from build123d import *

# Parameters (mm, degrees)
SKETCH_1_W          = 52
SKETCH_1_H          = 25
SKETCH_1_R          = 1.5
SKETCH_1_R_2        = 4
EXTRUDE_1_DEPTH     = 2
SKETCH_2_W          = 2
SKETCH_2_H          = 25
EXTRUDE_2_DEPTH     = 64.5
CUT_EXTRUDE_2_REACH = 91.001
SKETCH_3_R          = 1.5
FILLET_1_R          = 3


with BuildPart() as part:
    # 草图1 → 凸台-拉伸1 (new body)
    with BuildSketch(Plane(origin=(0, 0, 0), x_dir=(1, 0, 0), z_dir=(0, 1, 0))):
        with Locations((26, -12.5)):
            Rectangle(SKETCH_1_W, SKETCH_1_H)
        with Locations(Location((44.6, -12.5, 0), (0, 0, 270))):
            Circle(SKETCH_1_R, mode=Mode.SUBTRACT)
        with Locations(Location((26, -12.5, 0), (0, 0, 270))):
            Circle(SKETCH_1_R_2, mode=Mode.SUBTRACT)
        with Locations(Location((26, -19.5, 0), (0, 0, 270))):
            Circle(SKETCH_1_R, mode=Mode.SUBTRACT)
        with Locations(Location((19, -12.5, 0), (0, 0, 270))):
            Circle(SKETCH_1_R, mode=Mode.SUBTRACT)
        with Locations(Location((26, -5.5, 0), (0, 0, 270))):
            Circle(SKETCH_1_R, mode=Mode.SUBTRACT)
        with Locations(Location((33, -12.5, 0), (0, 0, 270))):
            Circle(SKETCH_1_R, mode=Mode.SUBTRACT)
        with Locations(Location((7.4, -12.5, 0), (0, 0, 90))):
            Circle(SKETCH_1_R, mode=Mode.SUBTRACT)
    extrude(amount=EXTRUDE_1_DEPTH)

    # 草图2 → 凸台-拉伸2 (add)
    with BuildSketch(Plane(origin=(0, 0, 0), x_dir=(1, 0, 0), z_dir=(0, 1, 0))):
        with Locations((-1, -12.5)):
            Rectangle(SKETCH_2_W, SKETCH_2_H)
        with Locations((53, -12.5)):
            Rectangle(SKETCH_2_W, SKETCH_2_H)
    extrude(amount=EXTRUDE_2_DEPTH)

    # 切除-拉伸2: up to this face of the body (flat: up to its plane)
    cut_extrude_2_end = Plane(part.part.faces().sort_by_distance((54, 32.25, 12.5))[0])
    # 草图3 → 切除-拉伸2 (cut, up to the picked face)
    with BuildSketch(Plane.ZY.offset(2), mode=Mode.PRIVATE) as cut_extrude_2_sk1:
        with BuildLine():
            Line((0, 64.5), (0, 52))
            ThreePointArc((0, 52), (3.661165235, 60.838834765), (12.5, 64.5))
            Line((12.5, 64.5), (0, 64.5))
        make_face()
    cut_extrude_2_tool1 = split(extrude(cut_extrude_2_sk1.sketch, amount=-CUT_EXTRUDE_2_REACH, mode=Mode.PRIVATE), bisect_by=cut_extrude_2_end, keep=Keep.BOTH, mode=Mode.PRIVATE)
    # 草图3 → 切除-拉伸2 (cut, up to the picked face)
    with BuildSketch(Plane.ZY.offset(2), mode=Mode.PRIVATE) as cut_extrude_2_sk2:
        with BuildLine():
            Line((25, 64.5), (12.5, 64.5))
            ThreePointArc((12.5, 64.5), (21.338834765, 60.838834765), (25, 52))
            Line((25, 52), (25, 64.5))
        make_face()
    cut_extrude_2_tool2 = split(extrude(cut_extrude_2_sk2.sketch, amount=-CUT_EXTRUDE_2_REACH, mode=Mode.PRIVATE), bisect_by=cut_extrude_2_end, keep=Keep.BOTH, mode=Mode.PRIVATE)
    # 草图3 → 切除-拉伸2 (cut, up to the picked face)
    with BuildSketch(Plane.ZY.offset(2), mode=Mode.PRIVATE) as cut_extrude_2_sk3:
        with BuildLine():
            ThreePointArc((16.5, 52), (12.5, 56), (8.5, 52))
            Line((8.5, 52), (16.5, 52))
        make_face()
    cut_extrude_2_tool3 = split(extrude(cut_extrude_2_sk3.sketch, amount=-CUT_EXTRUDE_2_REACH, mode=Mode.PRIVATE), bisect_by=cut_extrude_2_end, keep=Keep.BOTH, mode=Mode.PRIVATE)
    # 草图3 → 切除-拉伸2 (cut, up to the picked face)
    with BuildSketch(Plane.ZY.offset(2), mode=Mode.PRIVATE) as cut_extrude_2_sk4:
        with BuildLine():
            Line((16.5, 52), (8.5, 52))
            ThreePointArc((8.5, 52), (12.5, 48), (16.5, 52))
        make_face()
    cut_extrude_2_tool4 = split(extrude(cut_extrude_2_sk4.sketch, amount=-CUT_EXTRUDE_2_REACH, mode=Mode.PRIVATE), bisect_by=cut_extrude_2_end, keep=Keep.BOTH, mode=Mode.PRIVATE)
    # 草图3 → 切除-拉伸2 (cut, up to the picked face)
    with BuildSketch(Plane.ZY.offset(2), mode=Mode.PRIVATE) as cut_extrude_2_sk5:
        with BuildLine():
            ThreePointArc((16.5, 52), (12.5, 56), (8.5, 52))
            Line((8.5, 52), (16.5, 52))
        make_face()
    cut_extrude_2_tool5 = split(extrude(cut_extrude_2_sk5.sketch, amount=-CUT_EXTRUDE_2_REACH, mode=Mode.PRIVATE), bisect_by=cut_extrude_2_end, keep=Keep.BOTH, mode=Mode.PRIVATE)
    # 草图3 → 切除-拉伸2 (cut, up to the picked face)
    with BuildSketch(Plane.ZY.offset(2), mode=Mode.PRIVATE) as cut_extrude_2_sk6:
        with BuildLine():
            Line((16.5, 52), (8.5, 52))
            ThreePointArc((8.5, 52), (12.5, 48), (16.5, 52))
        make_face()
    cut_extrude_2_tool6 = split(extrude(cut_extrude_2_sk6.sketch, amount=-CUT_EXTRUDE_2_REACH, mode=Mode.PRIVATE), bisect_by=cut_extrude_2_end, keep=Keep.BOTH, mode=Mode.PRIVATE)
    # 草图3 → 切除-拉伸2 (cut, up to the picked face)
    with BuildSketch(Plane.ZY.offset(2), mode=Mode.PRIVATE) as cut_extrude_2_sk7:
        with Locations((12.5, 45)):
            Circle(SKETCH_3_R)
    cut_extrude_2_tool7 = split(extrude(cut_extrude_2_sk7.sketch, amount=-CUT_EXTRUDE_2_REACH, mode=Mode.PRIVATE), bisect_by=cut_extrude_2_end, keep=Keep.BOTH, mode=Mode.PRIVATE)
    # 草图3 → 切除-拉伸2 (cut, up to the picked face)
    with BuildSketch(Plane.ZY.offset(2), mode=Mode.PRIVATE) as cut_extrude_2_sk8:
        with Locations((12.5, 59)):
            Circle(SKETCH_3_R)
    cut_extrude_2_tool8 = split(extrude(cut_extrude_2_sk8.sketch, amount=-CUT_EXTRUDE_2_REACH, mode=Mode.PRIVATE), bisect_by=cut_extrude_2_end, keep=Keep.BOTH, mode=Mode.PRIVATE)
    # 草图3 → 切除-拉伸2 (cut, up to the picked face)
    with BuildSketch(Plane.ZY.offset(2), mode=Mode.PRIVATE) as cut_extrude_2_sk9:
        with Locations((5.5, 52)):
            Circle(SKETCH_3_R)
    cut_extrude_2_tool9 = split(extrude(cut_extrude_2_sk9.sketch, amount=-CUT_EXTRUDE_2_REACH, mode=Mode.PRIVATE), bisect_by=cut_extrude_2_end, keep=Keep.BOTH, mode=Mode.PRIVATE)
    # 草图3 → 切除-拉伸2 (cut, up to the picked face)
    with BuildSketch(Plane.ZY.offset(2), mode=Mode.PRIVATE) as cut_extrude_2_sk10:
        with Locations((19.5, 52)):
            Circle(SKETCH_3_R)
    cut_extrude_2_tool10 = split(extrude(cut_extrude_2_sk10.sketch, amount=-CUT_EXTRUDE_2_REACH, mode=Mode.PRIVATE), bisect_by=cut_extrude_2_end, keep=Keep.BOTH, mode=Mode.PRIVATE)
    add(cut_extrude_2_tool1.solids().sort_by(Axis((-2, 61.707901, 2.792099), (1, 0, 0)))[0], mode=Mode.SUBTRACT)
    add(cut_extrude_2_tool2.solids().sort_by(Axis((-2, 61.707901, 22.207901), (1, 0, 0)))[0], mode=Mode.SUBTRACT)
    add(cut_extrude_2_tool3.solids().sort_by(Axis((-2, 53.697653, 12.5), (1, 0, 0)))[0], mode=Mode.SUBTRACT)
    add(cut_extrude_2_tool4.solids().sort_by(Axis((-2, 50.302347, 12.5), (1, 0, 0)))[0], mode=Mode.SUBTRACT)
    add(cut_extrude_2_tool5.solids().sort_by(Axis((-2, 53.697653, 12.5), (1, 0, 0)))[0], mode=Mode.SUBTRACT)
    add(cut_extrude_2_tool6.solids().sort_by(Axis((-2, 50.302347, 12.5), (1, 0, 0)))[0], mode=Mode.SUBTRACT)
    add(cut_extrude_2_tool7.solids().sort_by(Axis((-2, 45, 12.5), (1, 0, 0)))[0], mode=Mode.SUBTRACT)
    add(cut_extrude_2_tool8.solids().sort_by(Axis((-2, 59, 12.5), (1, 0, 0)))[0], mode=Mode.SUBTRACT)
    add(cut_extrude_2_tool9.solids().sort_by(Axis((-2, 52, 5.5), (1, 0, 0)))[0], mode=Mode.SUBTRACT)
    add(cut_extrude_2_tool10.solids().sort_by(Axis((-2, 52, 19.5), (1, 0, 0)))[0], mode=Mode.SUBTRACT)

    # 圆角1
    fillet_1_edges = [part.edges().sort_by_distance(p)[0] for p in [
        (52, 2, 12.5),
        (0, 2, 12.5),
        (-2, 0, 12.5),
        (54, 0, 12.5),
    ]]
    fillet(fillet_1_edges, radius=FILLET_1_R)


solid = part.part
Geometry: final body of the model. Coordinates: model frame, mm. A direction names the side the tool comes from. Coordinates: 2 decimals unless noted, no trailing zeros. Write each loop counter-clockwise with the first axis right and the second up, starting at its lowest first coordinate (ties: lowest second). Pieces come first, ordered by that corner, then holes. Notation, with made-up numbers: (80, -17) - (138, -17) arc R17 cw to (138, 7) - close; hole circle Ø7 at (65.25, 81). An arc over 180 degrees is marked (long way). Return JSON: item names as keys, results as strings.
Item 1: Section query A-A (x = 26). Output: boundary loops of the cut face in (y, z), and give its area (3 significant figures).
Completed:
{"outline": "(0, 0) - (2, 0) - (2, 4) - (0, 4) - close; (0, 7) - (2, 7) - (2, 8.5) - (0, 8.5) - close; (0, 16.5) - (2, 16.5) - (2, 18) - (0, 18) - close; (0, 21) - (2, 21) - (2, 25) - (0, 25) - close", "area": "22.0 mm2"}
Item 2: Pull-direction query (Y, two-part tool) for faces 3 (the face through (-1, 51.1, 18.3)), 4 (the face through (27.487, 0.986, 5.305)), 5 (the face through (-1.14, 0.9, 12.32)); classes: +Y half, -Y half, draft (parallel to the pull), parting line (faces both ways), or undercut.
Completed:
{"face 3": "undercut", "face 4": "draft", "face 5": "-Y half"}
Item 3: Reachability of faces 1 (the face through (31, 2, 12)), 2 (the face through (26, 1, 25)) from +Z, -Z, +X, -X, +Y, -Y: full face, straight path, thin tool, end or side. Return the list, or none.
Completed:
{"face 1": "+Z, -Z, +Y", "face 2": "+Z, +X, -X, +Y, -Y"}
Item 4: Line query: L1, parallel to X at y = 26.5, z = 6.5; L2, parallel to Y at x = -1.1, z = 12.5; L3, parallel to X at y = 1.25, z = 12.5. Output: solid intervals per line, ascending.
Completed:
{"L1": "x = -2 to 0, 52 to 54", "L2": "y = 0.86 to 43.5, 46.5 to 48, 56 to 57.5, 60.5 to 64.5", "L3": "x = -1.44 to 5.9, 8.9 to 17.5, 20.5 to 22, 30 to 31.5, 34.5 to 43.1, 46.1 to 53.44"}
Item 5: Pin query (flat end, axial travel): pin 1 Ø10 at (x, y) = (7.5, 53) entering from -Z; pin 2 Ø4 at (x, z) = (13, 8.5) entering from +Y. Return the tip coordinate at first contact, or that it passes through.
Completed:
{"pin 1": "passes through", "pin 2": "stops at y = 2"}
Item 6: Section query C-C (x = 19). Output: boundary loops of the cut face in (y, z).
Completed:
{"outline": "(0, 0) - (2, 0) - (2, 11) - (0, 11) - close; (0, 14) - (2, 14) - (2, 25) - (0, 25) - close"}
Item 7: Section query B-B (y = 34). Output: boundary loops of the cut face in (x, z).
Completed:
{"outline": "(-2, 0) - (0, 0) - (0, 25) - (-2, 25) - close; (52, 0) - (54, 0) - (54, 25) - (52, 25) - close"}
Item 8: Section query D-D (z = 5.5). Output: boundary loops of the cut face in (x, y).
Completed:
{"outline": "(-2, 3) arc R3 ccw to (1, 0) - (24.5, 0) - (24.5, 2) - (3, 2) arc R3 cw to (0, 5) - (0, 50.5) - (-2, 50.5) - close; (-2, 53.5) - (0, 53.5) - (0, 62.36) - (-2, 62.36) - close; (27.5, 0) - (51, 0) arc R3 ccw to (54, 3) - (54, 50.5) - (52, 50.5) - (52, 5) arc R3 cw to (49, 2) - (27.5, 2) - close; (52, 53.5) - (54, 53.5) - (54, 62.36) - (52, 62.36) - close"}
